```python
from build123d import *

# Parameters (mm, degrees)
F1_DEPTH = 2
F2_R     = 15
F2_W     = 7.199677173
F2_H     = 2
F3_DEPTH = 3
F4_W     = 7.199677173
F4_H     = 2
F5_DEPTH = 2
F6_SIZE  = 1.99999
F7_W     = 7.199677173
F7_H     = 2
F8_DEPTH = 2
F9_SIZE  = 1.99999


# Not quite as in the source:
# - a fillet or chamfer that OpenCascade refuses, or shapes differently, is made with other operations: its cross-section is extruded or revolved along the edge and cut away or added
# - a fillet or chamfer is up to 0.001 mm smaller than in the source, because OpenCascade refuses the exact size


with BuildPart() as f1:
    # F0 (on Front) → F1 (new body)
    with BuildSketch(Plane.XZ):
        with BuildLine():
            ThreePointArc((-1.6914953012, 28.8060177118), (-2.3588223185, 28.5823009391), (-2.7564610355, 28.0015617609))
            Line((-2.7564610355, 28.0015617609), (-3.5831569694, 22.9014810175))
            Line((-3.5831569694, 22.9014810175), (-3.5831569694, 21.6677952558))
            ThreePointArc((-3.5831569694, 21.6677952558), (-2.8004223212, 19.8132576007), (-3.6002863199, 17.9660432041))
            Line((-3.6002863199, 17.9660432041), (-3.6002863199, 11.8300495669))
            Line((-3.6002863199, 11.8300495669), (3.5993908532, 11.8300495669))
            Line((3.5993908532, 11.8300495669), (3.5993908532, 17.969943583))
            ThreePointArc((3.5993908532, 17.969943583), (2.8023887863, 19.8030117696), (3.6017470993, 21.6350536793))
            Line((3.6017470993, 21.6350536793), (3.6017470993, 22.9016747326))
            Line((3.6017470993, 22.9016747326), (2.7295136824, 27.9675517231))
            ThreePointArc((2.7295136824, 27.9675517231), (2.3994359185, 28.5674317792), (1.7576538958, 28.8060177118))
            Line((1.7576538958, 28.8060177118), (-1.6914953012, 28.8060177118))
        make_face()
    extrude(amount=F1_DEPTH)

    # F2 (on face) → F3 (join)
    with BuildSketch(Plane(origin=(0, 0, 11.8300495669), x_dir=(1, 0, 0), z_dir=(0, 0, -1))):
        with Locations((0, 1)):
            Circle(F2_R)
        with Locations((-0.0004477333, 1)):
            Rectangle(F2_W, F2_H, mode=Mode.SUBTRACT)
        with Locations((-0.0004477333, 1)):
            Rectangle(F2_W, F2_H)
    extrude(amount=F3_DEPTH)

    # F4 (on face) → F5 (join)
    with BuildSketch(Plane(origin=(0, 0, 0), x_dir=(-1, 0, 0), z_dir=(0, 1, 0))):
        with Locations((0.0004477333, 12.8300495669)):
            Rectangle(F4_W, F4_H)
    extrude(amount=F5_DEPTH)

    # F6 (size 2 in the source; OpenCascade refuses exactly that, so slightly less here)
    f6_edges = [f1.edges().sort_by_distance(p)[0] for p in [
        (-0.000448, 2, 13.83005),
    ]]
    chamfer(f6_edges, length=F6_SIZE)

    # F7 (on face) → F8 (join)
    with BuildSketch(Plane.XZ.offset(2)):
        with Locations((-0.0004477333, 12.8300495669)):
            Rectangle(F7_W, F7_H)
    extrude(amount=F8_DEPTH)

    # F9 (size 2 in the source; OpenCascade refuses exactly that, so slightly less here)
    f9_edges = [f1.edges().sort_by_distance(p)[0] for p in [
        (-0.000448, -4, 13.83005),
    ]]
    chamfer(f9_edges, length=F9_SIZE)

    # F10: fillet of radius 5 on 1 edges, made by hand

    # F10_s1 → F10_t2 (revolve, cut)
    with BuildSketch(Plane.XZ.offset(1)):
        with BuildLine():
            ThreePointArc((15, 11.8300495669), (13.1560370926, 9.6467494343), (10.417424305, 8.8300495669))
            Line((10.417424305, 8.8300495669), (15, 8.8300495669))
            Line((15, 8.8300495669), (15, 11.8300495669))
        make_face()
    revolve(axis=Axis((0, -1, 8.8300495669), (0, 0, -1)), mode=Mode.SUBTRACT)


solid = f1.part
```
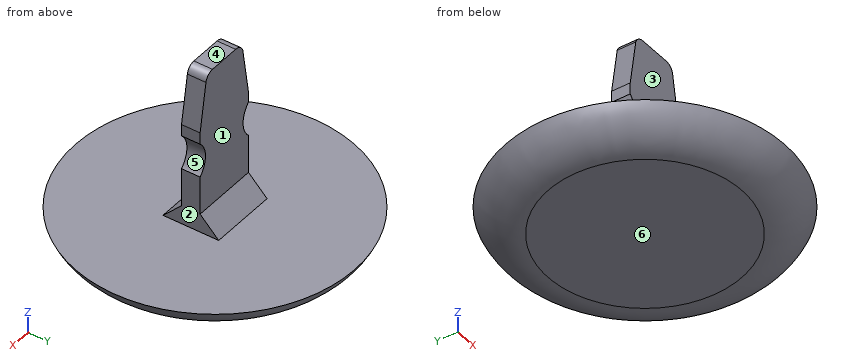
Here's how the part is built. I have some questions about the finished solid (model axes, mm). Face numbers are marked on the shaded views. A direction names the side the tool comes from. Coordinates: 2 decimals unless noted, no trailing zeros. Order: outer loops, then holes, each group sorted by start corner. A loop starts at its lowest first (then second) coordinate and runs counter-clockwise, first axis right, second up.
1) We'd pull the mould along Z, two halves only. Please class the marked faces 4, 5 and 6: +Z half, -Z half, draft (parallel to the pull), parting line (faces both ways), or undercut.
2) Which directions (+Z, -Z, +X, -X, +Y, -Y) give clear straight access to the entire face, cutting with the end or side of a thin tool? Please do the marked faces 1, 2 and 3.
3) Will these pins go through, and if not, where does the flat tip stop? pin 1 (3.5 mm diameter, centred on x = 1, z = 22, fed in from +Y); pin 2 (6 mm diameter, centred on y = -0.5, z = 21.5, fed in from -X); pin 3 (5 mm diameter, centred on x = 10.5, y = 6.5, fed in from -Z); pin 4 (0.6 mm diameter, centred on y = -1, z = 22.5, fed in from +X).
4) Imagine slicing it at B-B on z = 20.75. List the corners of the cut face in (x, y) for me.
5) Imagine slicing it at A-A on z = 17. List the corners of the cut face in (x, y) for me.
6) I need wall thicknesses on line 1 (Y direction, x = -1.5, z = 18.5); line 2 (X direction, y = -0.75, z = 14.25); line 3 (Z direction, x = -0.75, y = 2.5). Which ranges of each line are inside material? Lowest first, please.
Response values:
1. face 4: +Z half
1. face 5: undercut
1. face 6: -Z half
2. face 1: +Z, +X, -X, +Y
2. face 2: +Z, +X, +Y, -Y
2. face 3: +Z, +X, -X, -Y
3. pin 1: stops at y = 0
3. pin 2: stops at x = -3.58
3. pin 3: stops at z = 8.83
3. pin 4: stops at x = 3.6
4. outline: (-2.97, -2) - (2.99, -2) - (2.99, 0) - (-2.97, 0) - close
5. outline: (-3.6, -2) - (3.6, -2) - (3.6, 0) - (-3.6, 0) - close
6. line 1: y = -2 to 0
6. line 2: x = -3.6 to 3.6
6. line 3: z = 8.83 to 11.83
